from build123d import *

# Parameters (mm, degrees)
SKETCH2_R           = 1.95
SKETCH2_R_2         = 12.5
BOSS_EXTRUDE1_DEPTH = 3.175


with BuildPart() as part:
    # Sketch2 → Boss-Extrude1 (new body)
    with BuildSketch(Plane.XY):
        Polygon((-3.175, 0), (79.375, 0), (79.375, 12.7), (76.2, 12.7), (76.2, 14.375), (73.112, 14.375), (73.112, 12.625), (70.612, 12.625), (70.612, 14.375), (69.85, 14.375), (69.85, 17.375), (70.612, 17.375), (70.612, 19.125), (73.112, 19.125), (73.112, 17.375), (76.2, 17.375), (76.2, 27.075), (73.112, 27.075), (73.112, 25.325), (70.612, 25.325), (70.612, 27.075), (69.85, 27.075), (69.85, 30.075), (70.612, 30.075), (70.612, 31.825), (73.112, 31.825), (73.112, 30.075), (76.2, 30.075), (76.2, 31.75), (79.375, 31.75), (79.375, 44.45), (-3.175, 44.45), (-3.175, 31.75), (0, 31.75), (0, 30.075), (3.088, 30.075), (3.088, 31.825), (5.588, 31.825), (5.588, 30.075), (6.35, 30.075), (6.35, 27.075), (5.588, 27.075), (5.588, 25.325), (3.088, 25.325), (3.088, 27.075), (0, 27.075), (0, 17.375), (3.088, 17.375), (3.088, 19.125), (5.588, 19.125), (5.588, 17.375), (6.35, 17.375), (6.35, 14.375), (5.588, 14.375), (5.588, 12.625), (3.088, 12.625), (3.088, 14.375), (0, 14.375), (0, 12.7), (-3.175, 12.7), align=None)
        with Locations((22.6, 6.725)):
            Circle(SKETCH2_R, mode=Mode.SUBTRACT)
        with Locations((53.6, 6.725)):
            Circle(SKETCH2_R, mode=Mode.SUBTRACT)
        with Locations((38.1, 22.225)):
            Circle(SKETCH2_R_2, mode=Mode.SUBTRACT)
        with Locations((22.6, 37.725)):
            Circle(SKETCH2_R, mode=Mode.SUBTRACT)
        with Locations((53.6, 37.725)):
            Circle(SKETCH2_R, mode=Mode.SUBTRACT)
    extrude(amount=BOSS_EXTRUDE1_DEPTH)


solid = part.part
Can you work these out from the model? Positions are in its coordinate system, mm. A direction names the side the tool comes from. Give positions to 0.01 mm unless a question says otherwise; leave off trailing zeros. Order: outer loops, then holes, each group sorted by start corner. A loop starts at its lowest first (then second) coordinate and runs counter-clockwise, first axis right, second up. Notation, with made-up numbers: M -38,24 L 10,24 A20 cw 10,53 Z; hole C 58.5,55 d9. An arc over 180 degrees is marked long. Use one line per item in the form item = value. Start each with the question number.
Item 1: If we section it at C-C (y = 20): Write out the boundary of the cut face in (x, z) (3 decimals), then the cut area to 3 significant figures.
Item 2: If we section it at A-A (x = 38.1): Write out the boundary of the cut face in (y, z) (3 decimals), then the cut area to 3 significant figures.
Item 3: Will these pins go through, and if not, where does the flat tip stop? pin 1 Ø1.3 at (y, z) = (13.5, 1.5) entering from -X; pin 2 Ø0.9 at (y, z) = (13.5, 2.5) entering from +X; pin 3 Ø2.5 at (x, y) = (22.6, 37.725) entering from +Z.
Item 4: We'd pull the mould along X, two halves only. Please class faces 5 (the flat face through (75, 17.375, 2)), 6 (the flat face through (0, 14, 2)), 7 (the flat face through (3.088, 18, 2)): +X half, -X half, draft (parallel to the pull), parting line (faces both ways), or undercut.
Item 5: If I drill on line 1 along Y through (x, z) = (22.6, 0.7) (3 decimals); line 2 along Y through (x, z) = (72, 2.95) (3 decimals); line 3 along X through (y, z) = (13, 2.1) (3 decimals), over which ranges is the centre line in solid material (lowest first)?
Item 6: For faces 1 (the flat face through (73.112, 31, 2)), 2 (the flat face through (76.2, 14, 2)), 3 (the flat face through (6.35, 16, 2)), 4 (the flat face through (39, 44.45, 2)), which set-ups out of +Z, -Z, +X, -X, +Y, -Y let a thin tool reach every point of the face, with its end or its side?
Item 7: If we section it at B-B (x = 53.6): Write out the boundary of the cut face in (y, z) (3 decimals).
Item 8: If we section it at D-D (z = 2.1): State how many separate pieces and enclosed holes the cut face has, then the cut area to 3 significant figures.
Outcome:
q1.outline = M 0,0 L 25.8,0 L 25.8,3.175 L 0,3.175 Z; M 50.4,0 L 76.2,0 L 76.2,3.175 L 50.4,3.175 Z
q1.area = 164 mm2
q2.outline = M 0,0 L 9.725,0 L 9.725,3.175 L 0,3.175 Z; M 34.725,0 L 44.45,0 L 44.45,3.175 L 34.725,3.175 Z
q2.area = 61.8 mm2
q3.pin_1 = 0
q3.pin_2 = 76.2
q3.pin_3 = through
q4.face_5 = draft
q4.face_6 = -X half
q4.face_7 = undercut
q5.line_1 = 0 to 4.775, 8.675 to 35.775, 39.675 to 44.45
q5.line_2 = 0 to 12.625, 19.125 to 25.325, 31.825 to 44.45
q5.line_3 = 0 to 3.088, 5.588 to 29.665, 46.535 to 70.612, 73.112 to 76.2
q6.face_1 = +Z, -Z
q6.face_2 = +Z, -Z, +X
q6.face_3 = +Z, -Z, -X
q6.face_4 = +Z, -Z, +X, -X, +Y
q7.outline = M 0,0 L 4.775,0 L 4.775,3.175 L 0,3.175 Z; M 8.675,0 L 35.775,0 L 35.775,3.175 L 8.675,3.175 Z; M 39.675,0 L 44.45,0 L 44.45,3.175 L 39.675,3.175 Z
q8.separate_pieces = 1
q8.enclosed_holes = 5
q8.area = 2,900 mm2
